```python
from build123d import *

# Parameters (mm, degrees)
BOSS_EXTRUDE4_DEPTH = 6.35
SKETCH8_R           = 14.2875
SKETCH8_R_2         = 2.032
SKETCH8_R_3         = 9.525
CUT_EXTRUDE7_DEPTH  = 6.35
FILLET1_R           = 127
FILLET2_R           = 20.32
FILLET3_R           = 20.32
FILLET4_R           = 20.32
FILLET5_R           = 20.32
FILLET6_R           = 106.68
FILLET15_R          = 5.08
FILLET16_R          = 5.08
FILLET17_R          = 5.08
FILLET18_R          = 5.08


with BuildPart() as part:
    # Sketch6 → Boss-Extrude4 (new body)
    with BuildSketch(Plane.XY):
        Polygon((-430.595798314, -65.46403997), (-349.134252231, -52.10293935), (-114.184252231, -82.35181316), (-120.72454927, -133.15181316), (-347.342471816, -103.975661033), (-422.26372086, -116.26403997), align=None)
    extrude(amount=BOSS_EXTRUDE4_DEPTH)

    # Sketch8 → Cut-Extrude7 (cut)
    with BuildSketch(Plane.XY.offset(6.35)):
        with Locations((-406.219595957, -92.055134427)):
            Circle(SKETCH8_R)
        with Locations((-148.100562805, -105.64860282)):
            Circle(SKETCH8_R)
        with Locations((-364.383471272, -62.287100468)):
            Circle(SKETCH8_R_2)
        with Locations((-364.384308881, -98.101100468)):
            Circle(SKETCH8_R_2)
        with Locations((-328.570308884, -98.10061012)):
            Circle(SKETCH8_R_2)
        with Locations((-328.569471275, -62.28661013)):
            Circle(SKETCH8_R_2)
        with Locations((-346.476890078, -80.193855294)):
            Circle(SKETCH8_R_3)
        Polygon((-254.89844174, -115.877460566), (-253.367356027, -103.985163664), (-296.240101937, -98.465468917), (-297.77118765, -110.357765819), align=None)
    extrude(amount=-CUT_EXTRUDE7_DEPTH, mode=Mode.SUBTRACT)

    # Fillet1
    fillet1_edges = [part.edges().sort_by_distance(p)[0] for p in [
        (-349.134252231, -52.10293935, 3.175),
    ]]
    fillet(fillet1_edges, radius=FILLET1_R)

    # Fillet2
    fillet2_edges = [part.edges().sort_by_distance(p)[0] for p in [
        (-430.595798314, -65.46403997, 3.175),
    ]]
    fillet(fillet2_edges, radius=FILLET2_R)

    # Fillet3
    fillet3_edges = [part.edges().sort_by_distance(p)[0] for p in [
        (-422.26372086, -116.26403997, 3.175),
    ]]
    fillet(fillet3_edges, radius=FILLET3_R)

    # Fillet4
    fillet4_edges = [part.edges().sort_by_distance(p)[0] for p in [
        (-114.184252231, -82.35181316, 3.175),
    ]]
    fillet(fillet4_edges, radius=FILLET4_R)

    # Fillet5
    fillet5_edges = [part.edges().sort_by_distance(p)[0] for p in [
        (-120.72454927, -133.15181316, 3.175),
    ]]
    fillet(fillet5_edges, radius=FILLET5_R)

    # Fillet6
    fillet6_edges = [part.edges().sort_by_distance(p)[0] for p in [
        (-347.342471816, -103.975661033, 3.175),
    ]]
    fillet(fillet6_edges, radius=FILLET6_R)

    # Fillet15
    fillet15_edges = [part.edges().sort_by_distance(p)[0] for p in [
        (-254.89844174, -115.877460566, 3.175),
    ]]
    fillet(fillet15_edges, radius=FILLET15_R)

    # Fillet16
    fillet16_edges = [part.edges().sort_by_distance(p)[0] for p in [
        (-297.77118765, -110.357765819, 3.175),
    ]]
    fillet(fillet16_edges, radius=FILLET16_R)

    # Fillet17
    fillet17_edges = [part.edges().sort_by_distance(p)[0] for p in [
        (-296.240101937, -98.465468917, 3.175),
    ]]
    fillet(fillet17_edges, radius=FILLET17_R)

    # Fillet18
    fillet18_edges = [part.edges().sort_by_distance(p)[0] for p in [
        (-253.367356027, -103.985163664, 3.175),
    ]]
    fillet(fillet18_edges, radius=FILLET18_R)


solid = part.part
```
Geometry check sheet. Reference: the model listing, model coordinates, mm. A direction names the side the tool comes from. Give positions to 0.01 mm unless a question says otherwise; leave off trailing zeros. Order: outer loops, then holes, each group sorted by start corner. A loop starts at its lowest first (then second) coordinate and runs counter-clockwise, first axis right, second up.
1. Access from +Z, -Z, +X, -X, +Y, -Y to the whole of each face (thin tool, end or side, straight path). Record for faces 1 (the face through (-426.417, -90.939, 3.131)), 2 (the face through (-299.013, -108.658, 3.131)).
2. Section check C-C, the plane x = -271. Enter the section's corners in (y, z).
3. Section check B-B, the plane z = 3. Give the number of separate pieces and of enclosed holes in the cut face, and give its area (3 significant figures).
4. Section check A-A, the plane x = -157.5. Enter the section's corners in (y, z), and give its area (3 significant figures).
5. Gauge pin test, flat ends, axial feed: pin 1 Ø2 at (y, z) = (-87.5, 5.5) entering from +X; pin 2 Ø1.5 at (x, z) = (-267.5, 1) entering from +Y. Record the tip position at first contact, or that the pin passes through.
6. Thickness scan on L1, parallel to Y at x = -365.5, z = 1.75; L2, parallel to X at y = -85, z = 2.25; L3, parallel to Y at x = -389.5, z = 4.25. Record the ranges inside material, lowest first.
7. Release check for a two-part mould opening along Y. For faces 3 (the face through (-393.022, -97.527, 3.219)), 4 (the face through (-356, -80, 3)), 5 (the face through (-270, -92, 6.35)), 6 (the face through (-294.998, -100.166, 3.131)) record: pulls with the +Y half, pulls with the -Y half, needs draft (parallel to the pull), parting line crosses it, or undercut.
Values follow:
1. face 1: +Z, -Z, -X, -Y
1. face 2: +Z, -Z, -Y
2. outline: (-101.72, 0) - (-62.16, 0) - (-62.16, 6.35) - (-101.72, 6.35) - close
3. separate pieces: 1
3. enclosed holes: 7
3. area: 13,500 mm2
4. outline: (-128.42, 0) - (-116.41, 0) - (-116.41, 6.35) - (-128.42, 6.35) - close; (-94.89, 0) - (-76.78, 0) - (-76.78, 6.35) - (-94.89, 6.35) - close
4. area: 191 mm2
5. pin 1: stops at x = -120.12
5. pin 2: stops at y = -62.52
6. L1: y = -106.95 to -99.8, -96.4 to -63.98, -60.59 to -54.8
6. L2: x = -427.38 to -418.64, -393.8 to -354.7, -338.25 to -123.13
6. L3: y = -110.89 to -58.72
7. face 3: undercut
7. face 4: undercut
7. face 5: needs draft
7. face 6: pulls with the -Y half
